The model under review builds one solid part; all positions refer to its coordinate system, in mm. Face numbers are marked on the shaded views. A direction names the side the tool comes from. Round coordinates to 2 decimals unless told otherwise and drop trailing zeros. Loops run counter-clockwise (first coordinate to the right, second up) from the corner with the lowest first, then second, coordinate; pieces in that order, holes last. Notation, with made-up numbers: M -12.75,64.5 L 32.25,64.5 A23 ccw 32.25,75.5 Z; hole C 50.5,43 d9. An arc over 180 degrees is marked long. Answer as a JSON object with one key per item and string values. Group by question number.
Item 1: Consider section B-B (x = 0). Give the boundary of the cut face in (y, z) (3 decimals), and give its area (3 significant figures).
Item 2: The part is to be moulded in two halves that separate along Z. For the marked faces 4, 5, 6 and 7, say which applies: +Z half, -Z half, draft (parallel to the pull), parting line (faces both ways), or undercut.
Item 3: Consider section D-D (y = -3.75). Give the boundary of the cut face in (x, z) (3 decimals).
Item 4: Tool access review of the marked faces 1, 2 and 3: name each direction out of +Z, -Z, +X, -X, +Y, -Y from which nothing blocks a thin tool from reaching the whole face with its end or side.
Item 5: Consider section C-C (y = 1). Give the boundary of the cut face in (x, z), and give its area (3 significant figures).
Item 6: Consider section A-A (z = -4.45). Give the boundary of the cut face in (x, y).
Item 7: Insertion check: P1, Ø2.5, axis at x = 0.5, z = -3.5, coming from the -Y side; P2, Ø2.5, axis at x = 0.5, z = 4.5, coming from the -Y side; P3, Ø1.3, axis at y = 1, z = 1, coming from the -X side; P4, Ø1.5, axis at x = -1.5, y = 4.5, coming from the -Z side. Each pin has a flat end and moves straight along its axis. Give the tip position at first contact, or say it passes through.
Item 8: To check wall thickness, follow line 1 (X direction, y = 0.4, z = 4.45); line 2 (Y direction, x = -2, z = 2.25); line 3 (Z direction, x = -0.25, y = 0.25). State the ranges of each line that lie inside material, in increasing order.
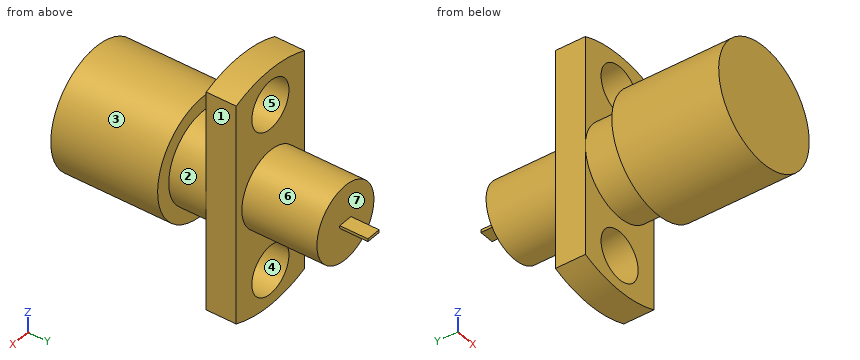
```python
from build123d import *

# Parameters (mm, degrees)
BOSS_EXTRUDE1_DEPTH = 1.6
SKETCH2_R           = 1.3
CUT_EXTRUDE1_DEPTH  = 1.6
SKETCH3_R           = 2
BOSS_EXTRUDE2_DEPTH = 4
BOSS_EXTRUDE3_DEPTH = 1.5
SKETCH5_R           = 2.4
BOSS_EXTRUDE5_DEPTH = 2
SKETCH6_R           = 3.175
BOSS_EXTRUDE7_DEPTH = 5.7


with BuildPart() as part:
    # Sketch1 → Boss-Extrude1 (new body)
    with BuildSketch(Plane(origin=(0, 0, 0), x_dir=(1, 0, 0), z_dir=(0, 1, 0))):
        with BuildLine():
            Line((-2.4, 5.878988008), (-2.4, -5.878988008))
            ThreePointArc((-2.4, -5.878988008), (0, -6.35), (2.4, -5.878988008))
            Line((2.4, -5.878988008), (2.4, 5.878988008))
            ThreePointArc((2.4, 5.878988008), (0, 6.35), (-2.4, 5.878988008))
        make_face()
    extrude(amount=BOSS_EXTRUDE1_DEPTH)

    # Sketch2 → Cut-Extrude1 (cut)
    with BuildSketch(Plane(origin=(0, 1.6, 0), x_dir=(1, 0, 0), z_dir=(0, 1, 0))):
        with Locations(Location((0, 4.45, 0), (0, 0, 270))):
            Circle(SKETCH2_R)
        with Locations(Location((0, -4.45, 0), (0, 0, 90))):
            Circle(SKETCH2_R)
    extrude(amount=-CUT_EXTRUDE1_DEPTH, mode=Mode.SUBTRACT)

    # Sketch3 → Boss-Extrude2 (add)
    with BuildSketch(Plane(origin=(0, 1.6, 0), x_dir=(1, 0, 0), z_dir=(0, 1, 0))):
        with Locations(Location((0, 0, 0), (0, 0, 90))):
            Circle(SKETCH3_R)
    extrude(amount=BOSS_EXTRUDE2_DEPTH)

    # Sketch4 → Boss-Extrude3 (add)
    with BuildSketch(Plane(origin=(0, 5.6, 0), x_dir=(1, 0, 0), z_dir=(0, 1, 0))):
        with BuildLine():
            Line((0.392905841, 0.075), (-0.392905841, 0.075))
            ThreePointArc((-0.392905841, 0.075), (-0.4, 0), (-0.392905841, -0.075))
            Line((-0.392905841, -0.075), (0.392905841, -0.075))
            ThreePointArc((0.392905841, -0.075), (0.4, 0), (0.392905841, 0.075))
        make_face()
    extrude(amount=BOSS_EXTRUDE3_DEPTH)

    # Sketch5 → Boss-Extrude5 (add)
    with BuildSketch(Plane.XZ):
        with Locations(Location((0, 0, 0), (0, 0, 180))):
            Circle(SKETCH5_R)
    extrude(amount=BOSS_EXTRUDE5_DEPTH)

    # Sketch6 → Boss-Extrude7 (add)
    with BuildSketch(Plane.XZ.offset(2)):
        with Locations(Location((0, 0, 0), (0, 0, 90))):
            Circle(SKETCH6_R)
    extrude(amount=BOSS_EXTRUDE7_DEPTH)


solid = part.part
```
Geometry results:
{
 "1": {"outline": "M -7.7,-3.175 L -2,-3.175 L -2,-2.4 L 0,-2.4 L 0,-3.15 L 1.6,-3.15 L 1.6,-2 L 5.6,-2 L 5.6,-0.075 L 7.1,-0.075 L 7.1,0.075 L 5.6,0.075 L 5.6,2 L 1.6,2 L 1.6,3.15 L 0,3.15 L 0,2.4 L -2,2.4 L -2,3.175 L -7.7,3.175 Z; M 0,-6.35 L 1.6,-6.35 L 1.6,-5.75 L 0,-5.75 Z; M 0,5.75 L 1.6,5.75 L 1.6,6.35 L 0,6.35 Z", "area": "74.0 mm^2"},
 "2": {"face 4": "undercut", "face 5": "undercut", "face 6": "parting line", "face 7": "draft"},
 "3": {"outline": "C 0,0 d6.35"},
 "4": {"face 1": "+Z, -Z, +X, +Y", "face 2": "none", "face 3": "-Y"},
 "5": {"outline": "M -2.4,-5.88 A6.35 ccw 2.4,-5.88 L 2.4,5.88 A6.35 ccw -2.4,5.88 Z; hole C 0,-4.45 d2.6; hole C 0,4.45 d2.6", "area": "48.9 mm^2"},
 "6": {"outline": "M -2.4,0 L -1.3,0 L -1.3,1.6 L -2.4,1.6 Z; M 1.3,0 L 2.4,0 L 2.4,1.6 L 1.3,1.6 Z"},
 "7": {"P1": "stops at y = -7.7", "P2": "stops at y = 0", "P3": "stops at x = -2.4", "P4": "stops at z = -1.85"},
 "8": {"line 1": "x = -2.4 to -1.3, 1.3 to 2.4", "line 2": "y = -7.7 to -2, 0 to 1.6", "line 3": "z = -6.35 to -5.73, -3.17 to 3.17, 5.73 to 6.35"}
}
